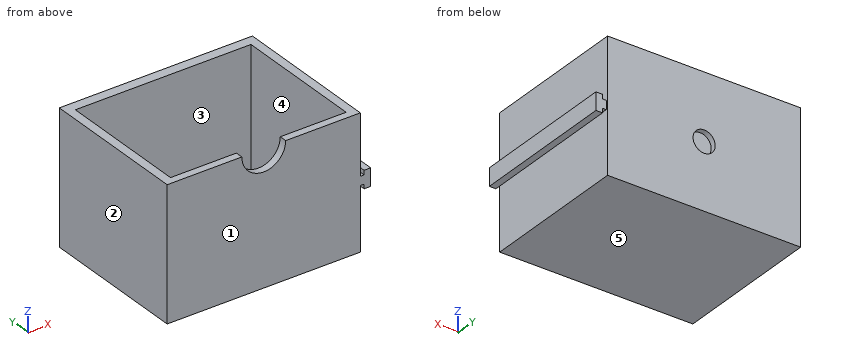
```python
from build123d import *

# Parameters (mm, degrees)
F0_W     = 55.88
F0_H     = 38.1
F1_DEPTH = 43.18
F2_W     = 50.8
F2_H     = 38.1
F3_DEPTH = 35.56
F4_R     = 6.35
F5_DEPTH = 25.4
F6_R     = 3.2
F7_DEPTH = 1.6002
F9_DEPTH = 42.672


with BuildPart() as f1:
    # F0 (on Front) → F1 (new body)
    with BuildSketch(Plane.XZ):
        with Locations((-20.484024, 19.05)):
            Rectangle(F0_W, F0_H)
    extrude(amount=-F1_DEPTH)

    # F2 (on face) → F3 (cut)
    with BuildSketch(Plane.XY.offset(38.1)):
        with Locations((-20.484024, 21.216264)):
            Rectangle(F2_W, F2_H)
    extrude(amount=-F3_DEPTH, mode=Mode.SUBTRACT)

    # F4 (on face) → F5 (cut)
    with BuildSketch(Plane.XZ):
        with Locations((-20.484024, 38.1)):
            Circle(F4_R)
    extrude(amount=-F5_DEPTH, mode=Mode.SUBTRACT)

    # F6 (on face) → F7 (cut)
    with BuildSketch(Plane(origin=(0, 43.18, 0), x_dir=(-1, 0, 0), z_dir=(0, 1, 0))):
        with Locations((20.484024, 19.05)):
            Circle(F6_R)
    extrude(amount=-F7_DEPTH, mode=Mode.SUBTRACT)

    # F8 (on face) → F9 (join)
    with BuildSketch(Plane.XZ):
        Polygon((8.556618, 22.011659), (8.556618, 20.741659), (7.455976, 20.741659), (7.455976, 18.201659), (8.556618, 18.201659), (8.556618, 16.931659), (10.461618, 16.931659), (10.461618, 22.011659), align=None)
    extrude(amount=-F9_DEPTH)


solid = f1.part
```
Check sheet for the modelled part. Datum: model origin and axes. Units: mm. Face numbers are marked on the shaded views. A direction names the side the tool comes from. Round coordinates to 2 decimals unless told otherwise and drop trailing zeros. Order: outer loops, then holes, each group sorted by start corner. A loop starts at its lowest first (then second) coordinate and runs counter-clockwise, first axis right, second up. Notation, with made-up numbers: (26.5, 39) - (81.5, 39) arc R19 ccw to (81.5, 54) - close; hole circle Ø1 at (40.5, -34.75). An arc over 180 degrees is marked (long way). Write item = value, one per line.
Q1. Go/stop test with flat-tipped pins: pin 1 (0.9 mm diameter, centred on x = 8, y = 31, fed in from -Z); pin 2 (1.5 mm diameter, centred on x = 9.5, z = 20.5, fed in from +Y); pin 3 (2 mm diameter, centred on x = 9.5, y = 29.5, fed in from -Z). Record where each tip stops, or that it passes through.
Computed:
pin_1 = 18.2
pin_2 = 42.67
pin_3 = 16.93
Q2. Section check A-A (z = 19.05). Record the boundary of the cut face in (x, y).
Computed:
outline = (-48.42, 0) - (10.46, 0) - (10.46, 42.67) - (7.46, 42.67) - (7.46, 43.18) - (-17.28, 43.18) - (-17.28, 41.58) - (-23.68, 41.58) - (-23.68, 43.18) - (-48.42, 43.18) - close; hole (-45.88, 2.17) - (4.92, 2.17) - (4.92, 40.27) - (-45.88, 40.27) - close
Q3. Section check B-B (x = 2.5). Record the boundary of the cut face in (y, z).
Computed:
outline = (0, 0) - (43.18, 0) - (43.18, 38.1) - (40.27, 38.1) - (40.27, 2.54) - (2.17, 2.54) - (2.17, 38.1) - (0, 38.1) - close
Q4. Section check C-C (y = 23). Record the boundary of the cut face in (x, z), and give its area (3 significant figures).
Computed:
outline = (-48.42, 0) - (7.46, 0) - (7.46, 18.2) - (8.56, 18.2) - (8.56, 16.93) - (10.46, 16.93) - (10.46, 22.01) - (8.56, 22.01) - (8.56, 20.74) - (7.46, 20.74) - (7.46, 38.1) - (4.92, 38.1) - (4.92, 2.54) - (-45.88, 2.54) - (-45.88, 38.1) - (-48.42, 38.1) - close
area = 335 mm^2
Q5. Thickness scan on line 1 along Y through (x, z) = (-10.5, 20); line 2 along X through (y, z) = (34.5, 21.5); line 3 along X through (y, z) = (34, 6). Record the ranges inside material, lowest first.
Computed:
line_1 = 0 to 2.17, 40.27 to 43.18
line_2 = -48.42 to -45.88, 4.92 to 7.46, 8.56 to 10.46
line_3 = -48.42 to -45.88, 4.92 to 7.46
Q6. Section check D-D (z = 12). Record the boundary of the cut face in (x, y).
Computed:
outline = (-48.42, 0) - (7.46, 0) - (7.46, 43.18) - (-48.42, 43.18) - close; hole (-45.88, 2.17) - (4.92, 2.17) - (4.92, 40.27) - (-45.88, 40.27) - close
Q7. Tool access check on the marked faces 4 and 5. Record the directions out of +Z, -Z, +X, -X, +Y, -Y that give a thin tool (end or side, any length) a straight path to the whole face; none if there is none.
Computed:
face_4 = +Z
face_5 = -Z, +X, -X, +Y, -Y
Q8. Draft check along X on the marked faces 1, 2 and 3. Enter one of: pulls with the +X half, pulls with the -X half, needs draft (parallel to the pull), parting line crosses it, or undercut.
Computed:
face_1 = needs draft
face_2 = pulls with the -X half
face_3 = undercut
